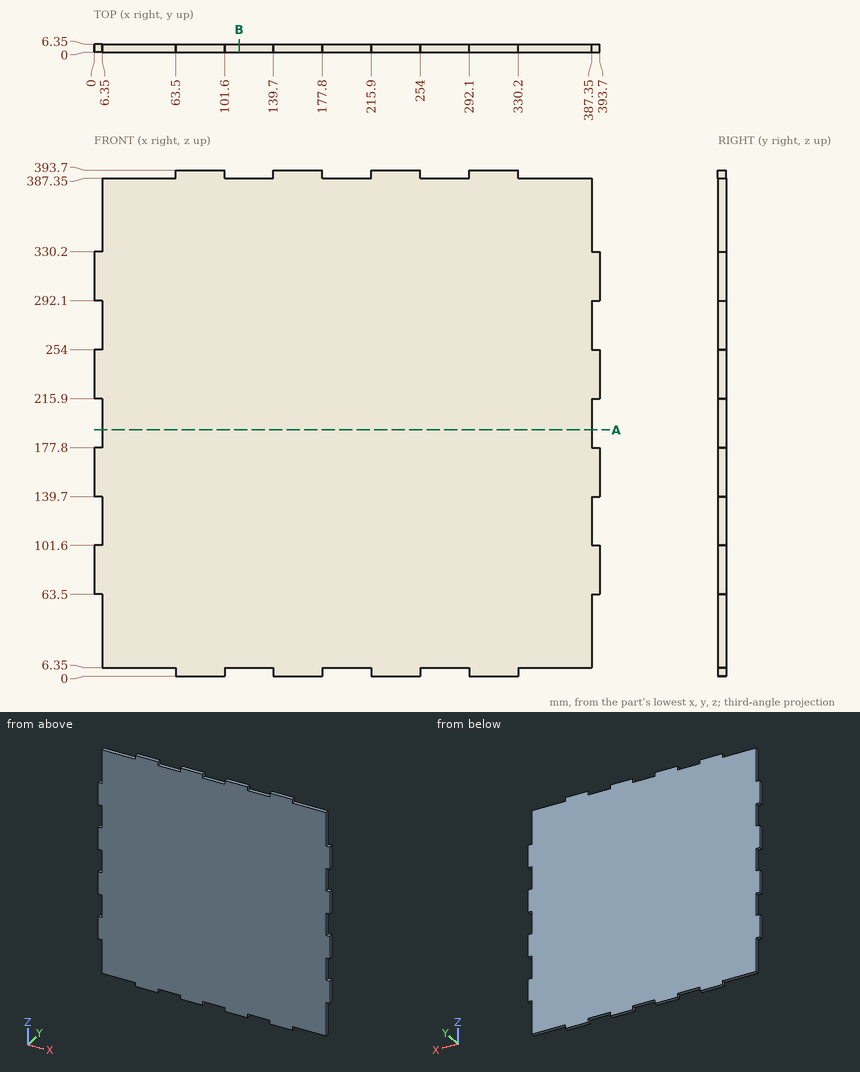
Drawing for the job (mm, zero at the part's lowest x, y, z). Give positions to 0.01 mm unless a question says otherwise; leave off trailing zeros. Order: outer loops, then holes, each group sorted by start corner. A loop starts at its lowest first (then second) coordinate and runs counter-clockwise, first axis right, second up. Notation, with made-up numbers: M 0.5,60 L 35.5,60 A24 ccw 35.5,92 Z; hole C -21,-30.5 d11. An arc over 180 degrees is marked long. Put each result on its own line as item: value. Start each with the question number.
(1) Flat gauge pins, fed straight in: pin 1 Ø3 at (x, y) = (346.5, 4) entering from +Z; pin 2 Ø3 at (y, z) = (4, 4) entering from +X; pin 3 Ø1.5 at (x, y) = (49, 2.5) entering from -Z. Where does each tip first touch, or does it go through?
(2) Saw through at B-B, the plane x = 113. Write the cut outline in (y, z), then the cut area to 3 significant figures.
(3) Saw through at A-A, the plane z = 191.5. Write the cut outline in (x, y), then the cut area to 3 significant figures.
(4) Drill centre line: line 1 along X through (y, z) = (5.5, 53). Where is it in solid material? Low to high.
Check result:
1. pin 1: stops at z = 387.35
1. pin 2: stops at x = 330.2
1. pin 3: stops at z = 6.35
2. outline: M 0,6.35 L 6.35,6.35 L 6.35,387.35 L 0,387.35 Z
2. area: 2,420 mm2
3. outline: M 6.35,0 L 387.35,0 L 387.35,6.35 L 6.35,6.35 Z
3. area: 2,420 mm2
4. line 1: x = 6.35 to 387.35
